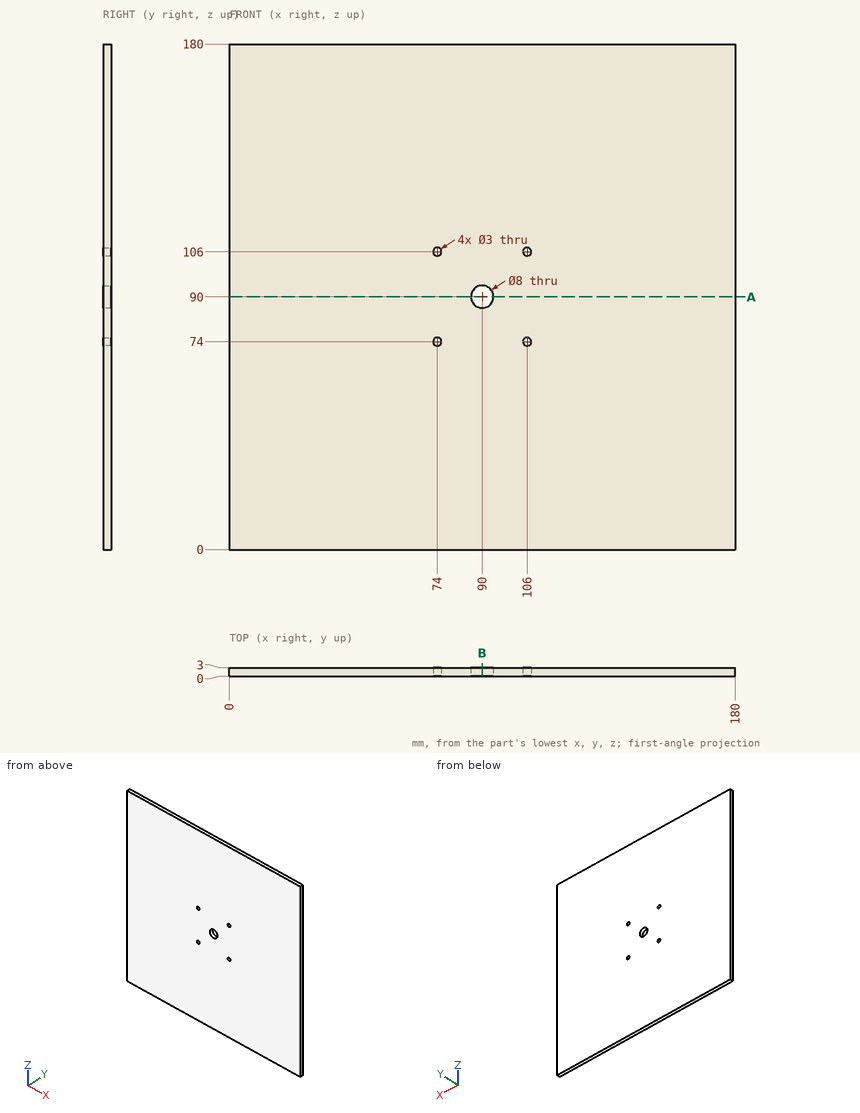
Job drawing, mm, ordinate dimensions from the low corner. One solid piece. Round coordinates to 2 decimals unless told otherwise and drop trailing zeros. Loops run counter-clockwise (first coordinate to the right, second up) from the corner with the lowest first, then second, coordinate; pieces in that order, holes last.
Item 1: Drop a flat-ended pin along its axis: P1, Ø1.8, axis at x = 106, z = 74, coming from the +Y side. Give the stop position or say it passes through.
Item 2: Cut at B-B, the plane x = 90. Give the cut face in (y, z).
Item 3: Drill centre lines: line 1 (Z direction, x = 106, y = 2.4); line 2 (Z direction, x = 106.5, y = 1.9). Where is each one in solid material? Low to high.
Item 4: Cut at A-A, the plane z = 90. Give the cut face in (x, y), then the cut area to 3 significant figures.
A:
1. P1: passes through
2. outline: (0, 0) - (3, 0) - (3, 86) - (0, 86) - close; (0, 94) - (3, 94) - (3, 180) - (0, 180) - close
3. line 1: z = 0 to 72.5, 75.5 to 104.5, 107.5 to 180
3. line 2: z = 0 to 72.59, 75.41 to 104.59, 107.41 to 180
4. outline: (0, 0) - (86, 0) - (86, 3) - (0, 3) - close; (94, 0) - (180, 0) - (180, 3) - (94, 3) - close
4. area: 516 mm2
